Geometry check sheet. Reference: the model listing, model coordinates, mm. Face numbers are marked on the shaded views. A direction names the side the tool comes from. Give positions to 0.01 mm unless a question says otherwise; leave off trailing zeros. Loops run counter-clockwise (first coordinate to the right, second up) from the corner with the lowest first, then second, coordinate; pieces in that order, holes last.
1. Cross-section at C-C, the plane x = 0. Record the cut outline in (y, z), plus the area to 3 significant figures.
2. Material ranges on L1, parallel to X at y = 92, z = -0.5; L2, parallel to Y at x = -4, z = 6.25; L3, parallel to Z at x = 0, y = 56, recorded low to high.
3. Cross-section at D-D, the plane z = -5.5. Record the cut outline in (x, y), plus the area to 3 significant figures.
4. Cross-section at A-A, the plane z = 0. Record the cut outline in (x, y), plus the area to 3 significant figures.
5. Cross-section at B-B, the plane y = 83. Record the cut outline in (x, z).
6. Go/stop test with flat-tipped pins: pin 1 Ø1.5 at (y, z) = (26, -1.5) entering from -X; pin 2 Ø1.3 at (y, z) = (11, -5.5) entering from -X; pin 3 Ø1.3 at (y, z) = (15.5, -5.5) entering from +X. Record where each tip stops, or that it passes through.
7. Tool access check on the marked faces 1 and 2. Record the directions out of +Z, -Z, +X, -X, +Y, -Y that give a thin tool (end or side, any length) a straight path to the whole face; none if there is none.
from build123d import *

# Parameters (mm, degrees)
SKETCH_2_W          = 7
SKETCH_2_H          = 7
CUT_EXTRUDE_1_DEPTH = 35
CUT_EXTRUDE_2_DEPTH = 3


with BuildPart() as part:
    # 草图1 → 旋转1 (revolve)
    with BuildSketch(Plane.XY):
        Polygon((0, 0), (-7, 0), (-7, 27), (-9, 27), (-9, 100), (0, 100), align=None)
    revolve(axis=Axis((0, 0, 0), (0, 1, 0)))

    # 草图2 → 切除-拉伸1 (cut)
    with BuildSketch(Plane(origin=(0, 100, 0), x_dir=(1, 0, 0), z_dir=(0, 1, 0))):
        Rectangle(SKETCH_2_W, SKETCH_2_H)
    extrude(amount=-CUT_EXTRUDE_1_DEPTH, mode=Mode.SUBTRACT)

    # 草图4 → 切除-拉伸2 (cut)
    with BuildSketch(Plane(origin=(0, 0, -7), x_dir=(-1, 0, 0), z_dir=(0, 0, -1))):
        with BuildLine():
            Line((-2.5, 4), (-2.5, 22))
            ThreePointArc((-2.5, 22), (0, 24.5), (2.5, 22))
            Line((2.5, 22), (2.5, 4))
            ThreePointArc((2.5, 4), (0, 1.5), (-2.5, 4))
        make_face()
    extrude(amount=-CUT_EXTRUDE_2_DEPTH, mode=Mode.SUBTRACT)


solid = part.part
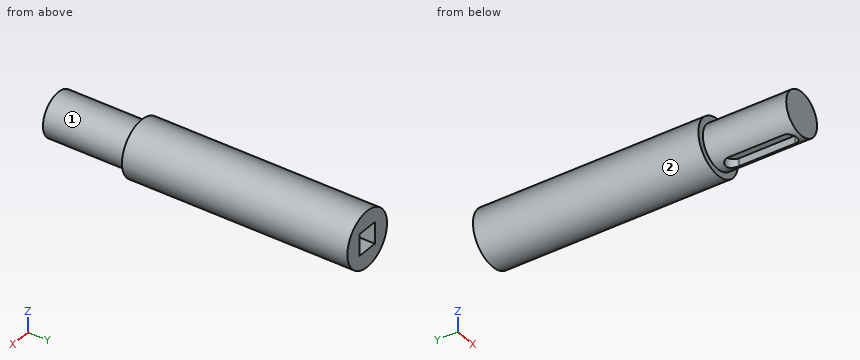
Result:
1. outline: (0, -7) - (1.5, -7) - (1.5, -4) - (24.5, -4) - (24.5, -7) - (27, -7) - (27, -9) - (100, -9) - (100, -3.5) - (65, -3.5) - (65, 3.5) - (100, 3.5) - (100, 9) - (27, 9) - (27, 7) - (0, 7) - close
1. area: 1,380 mm2
2. L1: x = -8.99 to -3.5, 3.5 to 8.99
2. L2: y = 27 to 100
2. L3: z = -9 to 9
3. outline: (-7.12, 27) - (-4.33, 27) - (-4.33, 0) - (4.33, 0) - (4.33, 27) - (7.12, 27) - (7.12, 100) - (-7.12, 100) - close; hole (-2.5, 4) arc R2.5 ccw to (2.5, 4) - (2.5, 22) arc R2.5 ccw to (-2.5, 22) - close
3. area: 1,160 mm2
4. outline: (-9, 27) - (-7, 27) - (-7, 0) - (7, 0) - (7, 27) - (9, 27) - (9, 100) - (3.5, 100) - (3.5, 65) - (-3.5, 65) - (-3.5, 100) - (-9, 100) - close
4. area: 1,450 mm2
5. outline: circle Ø18 at (0, 0); hole (-3.5, -3.5) - (3.5, -3.5) - (3.5, 3.5) - (-3.5, 3.5) - close
6. pin 1: stops at x = -6.96
6. pin 2: stops at x = -5.05
6. pin 3: stops at x = 5.05
7. face 1: -Y
7. face 2: +Y, -Y
